```python
from build123d import *

# Parameters (mm, degrees)
SKETCH_7_W          = 60
SKETCH_7_H          = 42
SKETCH_7_R          = 1.25
EXTRUDE_4_DEPTH     = 10
SKETCH_8_R          = 25
CUT_EXTRUDE_2_DEPTH = 50
SKETCH_9_R          = 5.5
EXTRUDE_5_DEPTH     = 4
CUT_EXTRUDE_4_DEPTH = 4
EXTRUDE_START       = -4
SKETCH_11_R         = 1.5
SKETCH_11_R_2       = 3
EXTRUDE_6_DEPTH     = 4
SKETCH_12_R         = 3
SKETCH_12_R_2       = 2.75
CUT_EXTRUDE_6_DEPTH = 2
SKETCH_15_R         = 1.25
CUT_EXTRUDE_7_DEPTH = 22
FILLET_1_R          = 2
FILLET_2_R          = 2
FILLET_3_R          = 2
FILLET_4_R          = 2
FILLET_6_R          = 2
FILLET_7_R          = 2


with BuildPart() as part:
    # 草图7 → 凸台-拉伸4 (new body)
    with BuildSketch(Plane.XY):
        with Locations((30, 21)):
            Rectangle(SKETCH_7_W, SKETCH_7_H)
        with Locations((2, 40)):
            Circle(SKETCH_7_R, mode=Mode.SUBTRACT)
        with Locations((2, 2)):
            Circle(SKETCH_7_R, mode=Mode.SUBTRACT)
        with Locations((58, 2)):
            Circle(SKETCH_7_R, mode=Mode.SUBTRACT)
        with Locations((58, 40)):
            Circle(SKETCH_7_R, mode=Mode.SUBTRACT)
    extrude(amount=EXTRUDE_4_DEPTH)

    # 草图8 → 切除-拉伸2 (cut)
    with BuildSketch(Plane.XZ):
        with Locations((25, 30)):
            Circle(SKETCH_8_R)
    extrude(amount=-CUT_EXTRUDE_2_DEPTH, mode=Mode.SUBTRACT)

    # 草图9 → 凸台-拉伸5 (add)
    with BuildSketch(Plane.XZ):
        with BuildLine():
            Line((0, 20), (0, 10))
            Line((0, 10), (10, 10))
            ThreePointArc((10, 10), (25, 5), (40, 10))
            Line((40, 10), (50, 10))
            Line((50, 10), (50, 20))
            Line((50, 20), (35, 20))
            ThreePointArc((35, 20), (25, 30), (15, 20))
            Line((15, 20), (0, 20))
        make_face()
        with Locations(Location((25, 20, 0), (0, 0, 270))):
            Circle(SKETCH_9_R, mode=Mode.SUBTRACT)
    extrude(amount=-EXTRUDE_5_DEPTH)

    # 草图10 → 切除-拉伸4 (cut)
    with BuildSketch(Plane.XZ):
        with BuildLine():
            ThreePointArc((0, 10), (8.660254038, 12.752551286), (14.142135624, 20))
            Line((14.142135624, 20), (0, 20))
            Line((0, 20), (0, 10))
        make_face()
        with BuildLine():
            Line((0, 20), (14.142135624, 20))
            ThreePointArc((14.142135624, 20), (14.783978395, 22.463470319), (15, 25))
            ThreePointArc((15, 25), (-10.606601718, 35.606601718), (0, 10))
            Line((0, 10), (0, 20))
        make_face()
        with BuildLine():
            ThreePointArc((65, 25), (47.463470319, 39.783978395), (35.857864376, 20))
            Line((35.857864376, 20), (50, 20))
            Line((50, 20), (50, 10))
            ThreePointArc((50, 10), (60.606601718, 14.393398282), (65, 25))
        make_face()
        with BuildLine():
            Line((50, 20), (35.857864376, 20))
            ThreePointArc((35.857864376, 20), (41.339745962, 12.752551286), (50, 10))
            Line((50, 10), (50, 20))
        make_face()
    extrude(amount=-CUT_EXTRUDE_4_DEPTH, mode=Mode.SUBTRACT)

    # 草图11 → 凸台-拉伸6 (add)
    with BuildSketch(Plane(origin=(0, 42, 0), x_dir=(1, 0, 0), z_dir=(0, 1, 0)).offset(EXTRUDE_START)):
        with BuildLine():
            ThreePointArc((40, -10), (25, -5), (10, -10))
            Line((10, -10), (0, -10))
            ThreePointArc((0, -10), (8.660254038, -12.752551286), (14.142135624, -20))
            Line((14.142135624, -20), (15, -20))
            ThreePointArc((15, -20), (25, -30), (35, -20))
            Line((35, -20), (35.857864376, -20))
            ThreePointArc((35.857864376, -20), (41.339745962, -12.752551286), (50, -10))
            Line((50, -10), (40, -10))
        make_face()
        with Locations(Location((25, -13, 0), (0, 0, 270))):
            Circle(SKETCH_11_R, mode=Mode.SUBTRACT)
        with Locations(Location((18, -20, 0), (0, 0, 270))):
            Circle(SKETCH_11_R, mode=Mode.SUBTRACT)
        with Locations(Location((25, -27, 0), (0, 0, 270))):
            Circle(SKETCH_11_R, mode=Mode.SUBTRACT)
        with Locations(Location((25, -20, 0), (0, 0, 270))):
            Circle(SKETCH_11_R_2, mode=Mode.SUBTRACT)
        with Locations(Location((32, -20, 0), (0, 0, 270))):
            Circle(SKETCH_11_R, mode=Mode.SUBTRACT)
    extrude(amount=EXTRUDE_6_DEPTH)

    # 草图12 → 切除-拉伸6 (cut)
    with BuildSketch(Plane(origin=(0, 42, 0), x_dir=(1, 0, 0), z_dir=(0, 1, 0))):
        with Locations(Location((25, -13, 0), (0, 0, 270))):
            Circle(SKETCH_12_R)
        with Locations(Location((18, -20, 0), (0, 0, 270))):
            Circle(SKETCH_12_R_2)
        with Locations(Location((25, -27, 0), (0, 0, 270))):
            Circle(SKETCH_12_R_2)
        with Locations(Location((32, -20, 0), (0, 0, 270))):
            Circle(SKETCH_12_R_2)
    extrude(amount=-CUT_EXTRUDE_6_DEPTH, mode=Mode.SUBTRACT)

    # 草图15 → 切除-拉伸7 (cut)
    with BuildSketch(Plane(origin=(0, 0, 0), x_dir=(-1, 0, 0), z_dir=(0, 0, -1))):
        with Locations((-2, 2)):
            Circle(SKETCH_15_R)
        with Locations((-2, 40)):
            Circle(SKETCH_15_R)
    extrude(amount=-CUT_EXTRUDE_7_DEPTH, mode=Mode.SUBTRACT)

    # 圆角1
    fillet_1_edges = [part.edges().sort_by_distance(p)[0] for p in [
        (0, 0, 5),
    ]]
    fillet(fillet_1_edges, radius=FILLET_1_R)

    # 圆角2
    fillet_2_edges = [part.edges().sort_by_distance(p)[0] for p in [
        (60, 0, 5),
    ]]
    fillet(fillet_2_edges, radius=FILLET_2_R)

    # 圆角3
    fillet_3_edges = [part.edges().sort_by_distance(p)[0] for p in [
        (60, 42, 5),
    ]]
    fillet(fillet_3_edges, radius=FILLET_3_R)

    # 圆角4
    fillet_4_edges = [part.edges().sort_by_distance(p)[0] for p in [
        (0, 42, 5),
    ]]
    fillet(fillet_4_edges, radius=FILLET_4_R)

    # 圆角6
    fillet_6_edges = [part.edges().sort_by_distance(p)[0] for p in [
        (40, 21, 10),
    ]]
    fillet(fillet_6_edges, radius=FILLET_6_R)

    # 圆角7
    fillet_7_edges = [part.edges().sort_by_distance(p)[0] for p in [
        (10, 21, 10),
    ]]
    fillet(fillet_7_edges, radius=FILLET_7_R)


solid = part.part
```
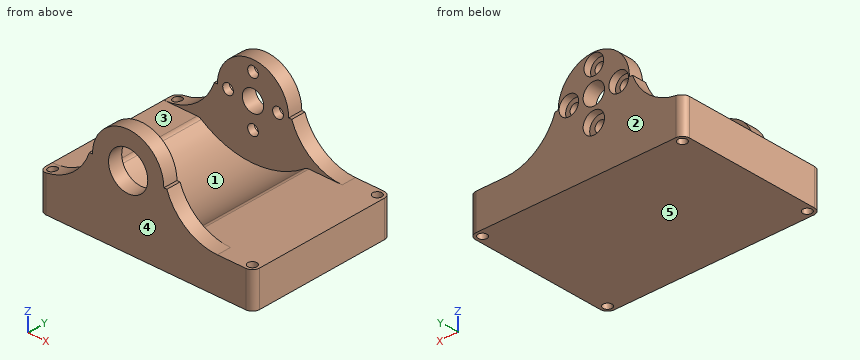
Geometry: final body of the model. Coordinates: model frame, mm. Face numbers are marked on the shaded views. A direction names the side the tool comes from. Round coordinates to 2 decimals unless told otherwise and drop trailing zeros. Loops run counter-clockwise (first coordinate to the right, second up) from the corner with the lowest first, then second, coordinate; pieces in that order, holes last.
Item 1: Section A-A, the plane z = 13. Output: boundary loops of the cut face in (x, y).
Checked values:
outline: (9, 0) - (41, 0) - (41, 4) - (9, 4) - close; (9, 38) - (23.5, 38) - (23.5, 40) - (22, 40) - (22, 42) - (9, 42) - close; (26.5, 38) - (41, 38) - (41, 42) - (28, 42) - (28, 40) - (26.5, 40) - close
Item 2: Section C-C, the plane x = 32. Output: boundary loops of the cut face in (y, z), plus the area to 3 significant figures.
Checked values:
outline: (0, 0) - (42, 0) - (42, 17.25) - (40, 17.25) - (40, 18.5) - (38, 18.5) - (38, 6) - (4, 6) - (4, 27.14) - (0, 27.14) - close; (38, 21.5) - (40, 21.5) - (40, 22.75) - (42, 22.75) - (42, 27.14) - (38, 27.14) - close
area: 404 mm2
Item 3: Section D-D, the plane z = 8. Output: boundary loops of the cut face in (x, y), plus the area to 3 significant figures.
Checked values:
outline: (0, 2) arc R2 ccw to (2, 0) - (58, 0) arc R2 ccw to (60, 2) - (60, 40) arc R2 ccw to (58, 42) - (2, 42) arc R2 ccw to (0, 40) - close; hole circle Ø2.5 at (2, 2); hole circle Ø2.5 at (2, 40); hole (13.13, 4) - (36.87, 4) - (36.87, 38) - (13.13, 38) - close; hole circle Ø2.5 at (58, 2); hole circle Ø2.5 at (58, 40)
area: 1,690 mm2
Item 4: Mould query, pull axis Y, two halves, no side actions, for the marked faces 3, 4 and 5. Classes: released by +Y, released by -Y, zero draft, split by the parting line, or undercut.
Checked values:
face 3: undercut
face 4: released by -Y
face 5: zero draft
Item 5: Contact query for flat-ended pins moving along their axis: P1, Ø12, axis at x = 39, y = 29, coming from the +Z side; P2, Ø8, axis at x = 33, y = 29.5, coming from the +Z side; P3, Ø0.7, axis at x = 14.5, y = 2, coming from the +Z side. Output: stop coordinate, or through.
Checked values:
P1: stops at z = 10
P2: stops at z = 8.07
P3: stops at z = 20
Item 6: Reachability of the marked faces 1 and 2 from +Z, -Z, +X, -X, +Y, -Y: full face, straight path, thin tool, end or side. Return the list, or none.
Checked values:
face 1: +Z
face 2: +Z, -Z, +X, -X, +Y
Item 7: Line query: L1, parallel to Y at x = 13, z = 13; L2, parallel to Y at x = 58, z = 2.5; L3, parallel to Y at x = 23, z = 15.5. Output: solid intervals per line, ascending.
Checked values:
L1: y = 0 to 4, 38 to 42
L2: y = 0 to 0.75, 3.25 to 38.75, 41.25 to 42
L3: y = 38 to 42
Item 8: Section B-B, the plane y = 11. Output: boundary loops of the cut face in (x, z), plus the area to 3 significant figures.
Checked values:
outline: (0, 0) - (60, 0) - (60, 10) - (40.65, 10) arc R2 ccw to (39.49, 9.63) arc R25 cw to (10.51, 9.63) arc R2 ccw to (9.35, 10) - (0, 10) - close
area: 498 mm2
